Check sheet for the modelled part. Datum: model origin and axes. Units: mm. Face numbers are marked on the shaded views. A direction names the side the tool comes from. Give positions to 0.01 mm unless a question says otherwise; leave off trailing zeros. Loops run counter-clockwise (first coordinate to the right, second up) from the corner with the lowest first, then second, coordinate; pieces in that order, holes last. Notation, with made-up numbers: (-21, 7.5) - (-11, 7.5) arc R10 cw to (-11, 26.5) - close; hole circle Ø7 at (11.5, -3.5). An arc over 180 degrees is marked (long way). Answer in a Markdown table with one row per item. Add a question column.
(1) Go/stop test with flat-tipped pins: P1, Ø5, axis at x = 0, z = -10, coming from the -Y side; P2, Ø2, axis at y = 0.5, z = 3.5, coming from the +X side (3 decimals); P3, Ø3, axis at x = -3.5, z = -5, coming from the -Y side; P4, Ø3, axis at x = -10, z = 0, coming from the +Y side. Record where each tip stops, or that it passes through.
(2) Sectioned sample at D-D on y = 1.25. Enter the section's corners in (x, z), then the cut area to 3 significant figures.
(3) Draft check along Z on the marked faces 1 and 2. Enter one of: released by +Z, released by -Z, zero draft, split by the parting line, or undercut.
(4) Sectioned sample at C-C on x = 10. Enter the section's corners in (y, z), then the cut area to 3 significant figures.
(5) Set-up check for the marked faces 3, 4 and 5: record each of +Z, -Z, +X, -X, +Y, -Y from which the full face is reachable in a straight line by a thin tool's end or side.
(6) Sectioned sample at B-B on y = -5.25. Enter the section's corners in (x, z).
(7) Sectioned sample at A-A on z = 0. Enter the section's corners in (x, y) (3 decimals), then the cut area to 3 significant figures.
(8) Thickness scan on L1, parallel to X at y = -0.7, z = 0 (3 decimals); L2, parallel to X at y = 1.8, z = 0; L3, parallel to Y at x = -3.5, z = -12. Record the ranges inside material, lowest first.
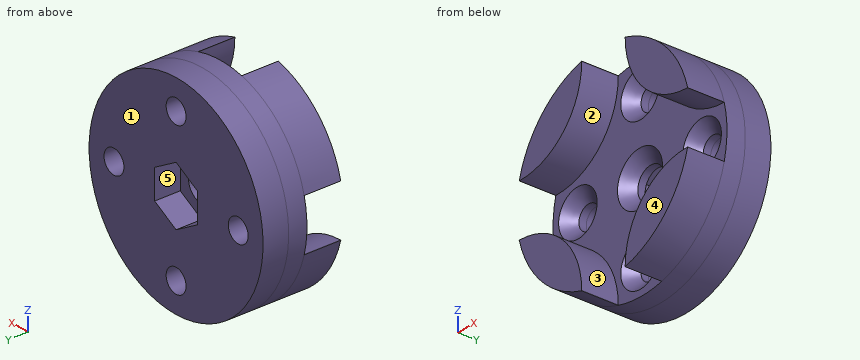
from build123d import *

# Parameters (mm, degrees)
SKETCH1_R           = 14
SKETCH1_R_2         = 1.6
BOSS_EXTRUDE1_DEPTH = 3.5
BOSS_EXTRUDE2_START = 2.5
SKETCH2_R           = 14
SKETCH2_R_2         = 2.125
SKETCH2_R_3         = 1.6
BOSS_EXTRUDE2_DEPTH = 2.5
CHAMFER1_SIZE       = 1.5
BOSS_EXTRUDE3_START = 5
BOSS_EXTRUDE3_DEPTH = 5
FILLET1_R           = 10


with BuildPart() as part:
    # Sketch1 → Boss-Extrude1 (new body)
    with BuildSketch(Plane(origin=(0, 0, 0), x_dir=(1, 0, 0), z_dir=(0, 1, 0))):
        with Locations(Location((0, 0, 0), (0, 0, 270))):
            Circle(SKETCH1_R)
        with Locations(Location((0, 10, 0), (0, 0, 270))):
            Circle(SKETCH1_R_2, mode=Mode.SUBTRACT)
        with Locations(Location((10, 0, 0), (0, 0, 270))):
            Circle(SKETCH1_R_2, mode=Mode.SUBTRACT)
        with Locations(Location((0, -10, 0), (0, 0, 270))):
            Circle(SKETCH1_R_2, mode=Mode.SUBTRACT)
        with Locations(Location((-10, 0, 0), (0, 0, 270))):
            Circle(SKETCH1_R_2, mode=Mode.SUBTRACT)
        Polygon((0, 3.983716857), (-3.45, 1.991858429), (-3.45, -1.991858429), (0, -3.983716857), (3.45, -1.991858429), (3.45, 1.991858429), align=None, mode=Mode.SUBTRACT)
    extrude(amount=BOSS_EXTRUDE1_DEPTH)

    # Sketch2 → Boss-Extrude2 (add)
    with BuildSketch(Plane.XZ.offset(BOSS_EXTRUDE2_START)):
        with Locations(Location((0, 0, 0), (0, 0, 270))):
            Circle(SKETCH2_R)
        with Locations(Location((0, 0, 0), (0, 0, 270))):
            Circle(SKETCH2_R_2, mode=Mode.SUBTRACT)
        with Locations(Location((10, 0, 0), (0, 0, 270))):
            Circle(SKETCH2_R_3, mode=Mode.SUBTRACT)
        with Locations(Location((0, -10, 0), (0, 0, 270))):
            Circle(SKETCH2_R_3, mode=Mode.SUBTRACT)
        with Locations(Location((-10, 0, 0), (0, 0, 270))):
            Circle(SKETCH2_R_3, mode=Mode.SUBTRACT)
        with Locations(Location((0, 10, 0), (0, 0, 270))):
            Circle(SKETCH2_R_3, mode=Mode.SUBTRACT)
    extrude(amount=-BOSS_EXTRUDE2_DEPTH)

    # Chamfer1
    chamfer1_edges = [part.edges().sort_by_distance(p)[0] for p in [
        (0, -2.5, 2.125),
        (10, -2.5, 1.6),
        (0, -2.5, -8.4),
        (-10, -2.5, 1.6),
        (0, -2.5, 11.6),
    ]]
    chamfer(chamfer1_edges, length=CHAMFER1_SIZE)

    # Sketch3 → Boss-Extrude3 (add)
    with BuildSketch(Plane.XZ.offset(2.5).offset(BOSS_EXTRUDE3_START)):
        with BuildLine():
            ThreePointArc((-3.5, 13.555441712), (-9.899494937, 9.899494937), (-13.555441712, 3.5))
            Line((-13.555441712, 3.5), (-4, 3.5))
            Line((-4, 3.5), (-3.5, 3.5))
            Line((-3.5, 3.5), (-3.5, 4))
            Line((-3.5, 4), (-3.5, 13.555441712))
        make_face()
        with BuildLine():
            Line((4, 3.5), (13.555441712, 3.5))
            ThreePointArc((13.555441712, 3.5), (9.899494937, 9.899494937), (3.5, 13.555441712))
            Line((3.5, 13.555441712), (3.5, 4))
            Line((3.5, 4), (3.5, 3.5))
            Line((3.5, 3.5), (4, 3.5))
        make_face()
        with BuildLine():
            Line((13.555441712, -3.5), (4, -3.5))
            Line((4, -3.5), (3.5, -3.5))
            Line((3.5, -3.5), (3.5, -4))
            Line((3.5, -4), (3.5, -13.555441712))
            ThreePointArc((3.5, -13.555441712), (9.899494937, -9.899494937), (13.555441712, -3.5))
        make_face()
        with BuildLine():
            ThreePointArc((-13.555441712, -3.5), (-9.899494937, -9.899494937), (-3.5, -13.555441712))
            Line((-3.5, -13.555441712), (-3.5, -4))
            Line((-3.5, -4), (-3.5, -3.5))
            Line((-3.5, -3.5), (-4, -3.5))
            Line((-4, -3.5), (-13.555441712, -3.5))
        make_face()
    extrude(amount=-BOSS_EXTRUDE3_DEPTH)

    # Fillet1
    fillet1_edges = [part.edges().sort_by_distance(p)[0] for p in [
        (-3.5, -5, 3.5),
        (-3.5, -5, -3.5),
        (3.5, -5, -3.5),
        (3.5, -5, 3.5),
    ]]
    fillet(fillet1_edges, radius=FILLET1_R)


solid = part.part
Reply:
| question | item | result |
|---|---|---|
| 1 | P1 | y = -1.9 |
| 1 | P2 | x = 13.775 |
| 1 | P3 | y = -2.5 |
| 1 | P4 | through |
| 2 | outline | circle Ø28 at (0, 0); hole circle Ø3.2 at (-10, 0); hole (-3.45, -1.99) - (0, -3.98) - (3.45, -1.99) - (3.45, 1.99) - (0, 3.98) - (-3.45, 1.99) - close; hole circle Ø3.2 at (0, -10); hole circle Ø3.2 at (0, 10); hole circle Ø3.2 at (10, 0) |
| 2 | area | 542 mm^2 |
| 3 | face 1 | zero draft |
| 3 | face 2 | undercut |
| 4 | outline | (-7.5, -9.8) - (3.5, -9.8) - (3.5, -1.6) - (-1, -1.6) - (-2.5, -3.1) - (-2.5, -4.13) - (-7.5, -4.13) - close; (-7.5, 4.13) - (-2.5, 4.13) - (-2.5, 3.1) - (-1, 1.6) - (3.5, 1.6) - (3.5, 9.8) - (-7.5, 9.8) - close |
| 4 | area | 153 mm^2 |
| 5 | face 3 | -Y |
| 5 | face 4 | +Z, -Z, +X, -X, -Y |
| 5 | face 5 | +Y |
| 6 | outline | (-13.56, -3.5) arc R14 ccw to (-3.5, -13.56) - (-3.5, -13.5) arc R10 ccw to (-13.5, -3.5) - close; (-13.56, 3.5) - (-13.5, 3.5) arc R10 ccw to (-3.5, 13.5) - (-3.5, 13.56) arc R14 ccw to start; (3.5, -13.56) arc R14 ccw to (13.56, -3.5) - (13.5, -3.5) arc R10 ccw to (3.5, -13.5) - close; (3.5, 13.5) arc R10 ccw to (13.5, 3.5) - (13.56, 3.5) arc R14 ccw to (3.5, 13.56) - close |
| 7 | outline | (-14, -2.5) - (-13.1, -2.5) - (-11.6, -1) - (-11.6, 3.5) - (-14, 3.5) - close; (-8.4, -1) - (-6.9, -2.5) - (-3.625, -2.5) - (-2.125, -1) - (-2.125, 0) - (-3.45, 0) - (-3.45, 3.5) - (-8.4, 3.5) - close; (2.125, -1) - (3.625, -2.5) - (6.9, -2.5) - (8.4, -1) - (8.4, 3.5) - (3.45, 3.5) - (3.45, 0) - (2.125, 0) - close; (11.6, -1) - (13.1, -2.5) - (14, -2.5) - (14, 3.5) - (11.6, 3.5) - close |
| 7 | area | 88.1 mm^2 |
| 8 | L1 | -14 to -11.6, -8.4 to -2.125, 2.125 to 8.4, 11.6 to 14 |
| 8 | L2 | -14 to -11.6, -8.4 to -3.45, 3.45 to 8.4, 11.6 to 14 |
| 8 | L3 | -2.5 to 3.5 |
